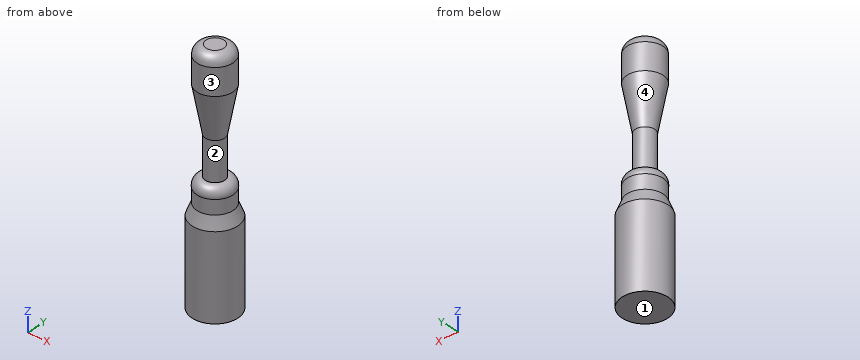
```python
from build123d import *


with BuildPart() as f1:
    # F0 (on Front) → F1 (revolve)
    with BuildSketch(Plane.XZ):
        with BuildLine():
            Line((3.672682, 0), (0, 0))
            Line((0, 0), (0, -100))
            Line((0, -100), (9.5, -100))
            Line((9.5, -100), (9.5, -65))
            Line((9.5, -65), (7.5, -60))
            Line((7.5, -60), (7.5, -54.091204))
            ThreePointArc((7.5, -54.091204), (6.709919, -51.224397), (4, -50))
            Line((4, -50), (4, -34))
            Line((4, -34), (7.5, -15))
            Line((7.5, -15), (7.5, -3.996271))
            ThreePointArc((7.5, -3.996271), (6.388834, -1.22957), (3.672682, 0))
        make_face()
    revolve(axis=Axis((0, 0, -50), (0, 0, 1)))


solid = f1.part
```
Input: part model. Units: mm. Frame: model coordinates. Face numbers are marked on the shaded views. Give positions to 0.01 mm unless a question says otherwise; leave off trailing zeros. Order: outer loops, then holes, each group sorted by start corner. A loop starts at its lowest first (then second) coordinate and runs counter-clockwise, first axis right, second up.
1. Draft query along Z for the marked faces 1, 2, 3 and 4. Return one class per face: released by +Z, released by -Z, zero draft, split by the parting line, or undercut.
Computed:
face 1: released by -Z
face 2: undercut
face 3: zero draft
face 4: undercut
2. Cut plane A-A (z = -81). Return loops of the section in (x, y), and give its area (3 significant figures).
Computed:
outline: circle Ø19 at (0, 0)
area: 284 mm2
3. Line query: probe 1 along Y at (x, z) = (2.5, -61); probe 2 along Z at (x, y) = (6.75, -4.25); probe 3 along Z at (x, y) = (7.5, 4.75). Output: solid intervals per line, ascending.
Computed:
probe 1: y = -7.49 to 7.49
probe 2: z = -100 to -61.19
probe 3: z = -100 to -63.44
4. Cut plane B-B (z = -52.5). Return loops of the section in (x, y).
Computed:
outline: circle Ø14.81 at (0, 0)
5. Pin query (flat end, axial travel): pin 1 Ø10 at (y, z) = (-3, -66.5) entering from -X; pin 2 Ø5 at (x, z) = (3, -24.5) entering from -Y; pin 3 Ø10 at (x, z) = (3, -40) entering from -Y; pin 4 Ø1.5 at (x, z) = (-6.5, -60.5) entering from +Y. Return the tip coordinate at first contact, or that it passes through.
Computed:
pin 1: stops at x = -9.5
pin 2: stops at y = -5.95
pin 3: stops at y = -4
pin 4: stops at y = 5.23
